The drawing under review shows one solid part. Ordinate dimensions are in mm from its lowest x, y, z. Round coordinates to 2 decimals unless told otherwise and drop trailing zeros. Write each loop counter-clockwise with the first axis right and the second up, starting at its lowest first coordinate (ties: lowest second). Pieces come first, ordered by that corner, then holes. Notation, with made-up numbers: (28, 39.5) -> (40, 39.5) arc R12 ccw to (40, 53.5) -> close; hole circle Ø10 at (-17, 47). An arc over 180 degrees is marked (long way). Write item = value, one per line. Start each with the question number.
Item 1: Add section C-C, the plane z = 32.5. State the section outline as (x, y) points.
Item 2: To check wall thickness, follow L1, parallel to Z at x = 18.5, y = 6.9; L2, parallel to X at y = 7, z = 7; L3, parallel to Y at x = 14, z = 21.5. State the ranges of each line that lie inside material, in increasing order.
Item 3: For pin 1 Ø5 at (x, z) = (18.5, 32.5) entering from +Y; pin 2 Ø2.5 at (x, z) = (14.5, 18.5) entering from -Y; pin 3 Ø0.9 at (x, z) = (8, 7.5) entering from +Y, all flat-tipped, find the tip position at first contact; note any pin that passes through.
Item 4: Mouldability with a two-part tool opening along X and no side actions: class the marked faces 1, 2 and 3 as released by +X, released by -X, zero draft, split by the parting line, or undercut.
Item 5: Add section A-A, the plane y = 0.5. State the section outline as (x, z) points, then the cut area to 3 significant figures.
Item 6: Add section D-D, the plane z = 10. State the section outline as (x, y) points, then the cut area to 4 significant figures.
Item 7: Add section B-B, the plane x = 18.5. State the section outline as (y, z) points.
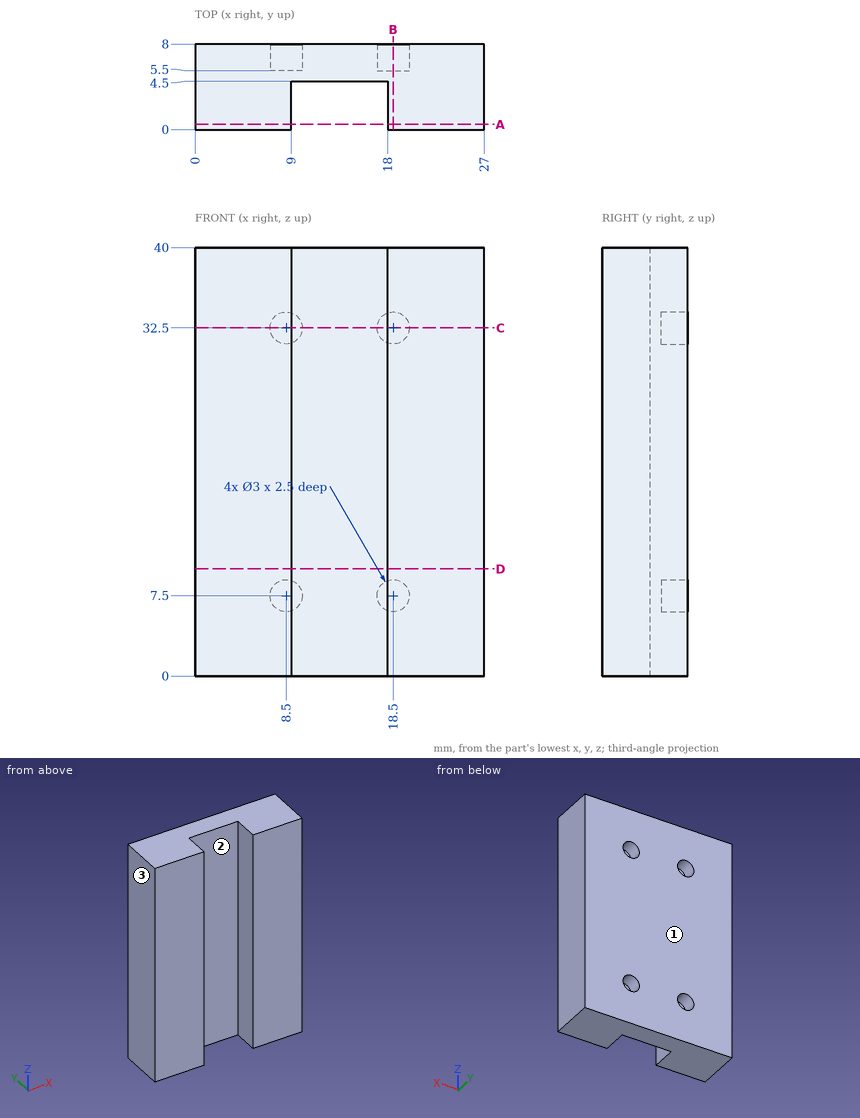
Result set:
q1.outline = (0, 0) -> (9, 0) -> (9, 4.5) -> (18, 4.5) -> (18, 0) -> (27, 0) -> (27, 8) -> (20, 8) -> (20, 5.5) -> (17, 5.5) -> (17, 8) -> (10, 8) -> (10, 5.5) -> (7, 5.5) -> (7, 8) -> (0, 8) -> close
q2.L1 = 0 to 6, 9 to 31, 34 to 40
q2.L2 = 0 to 7.09, 9.91 to 17.09, 19.91 to 27
q2.L3 = 4.5 to 8
q3.pin_1 = 8
q3.pin_2 = 4.5
q3.pin_3 = 5.5
q4.face_1 = zero draft
q4.face_2 = undercut
q4.face_3 = released by -X
q5.outline = (0, 0) -> (9, 0) -> (9, 40) -> (0, 40) -> close; (18, 0) -> (27, 0) -> (27, 40) -> (18, 40) -> close
q5.area = 720 mm²
q6.outline = (0, 0) -> (9, 0) -> (9, 4.5) -> (18, 4.5) -> (18, 0) -> (27, 0) -> (27, 8) -> (0, 8) -> close
q6.area = 175.5 mm²
q7.outline = (0, 0) -> (8, 0) -> (8, 6) -> (5.5, 6) -> (5.5, 9) -> (8, 9) -> (8, 31) -> (5.5, 31) -> (5.5, 34) -> (8, 34) -> (8, 40) -> (0, 40) -> close
